Could you check a few things on this model? Use its own coordinates, in mm. A direction names the side the tool comes from. Round coordinates to 2 decimals unless told otherwise and drop trailing zeros. Order: outer loops, then holes, each group sorted by start corner. A loop starts at its lowest first (then second) coordinate and runs counter-clockwise, first axis right, second up. Notation, with made-up numbers: M 26,30 L 73,30 A18 ccw 73,45 Z; hole C -32,14.25 d11. An arc over 180 degrees is marked long. Write each question's results on one line, items separated by ' | '. Start each with the question number.
1. Suppose I cut it at A-A on z = 1.75. Write out the boundary of the cut face in (x, y).
2. Suppose I cut it at B-B on x = -16. Write out the boundary of the cut face in (y, z).
3. Suppose I cut it at C-C on y = 9. Write out the boundary of the cut face in (x, z), and give its area (3 significant figures).
4. Please list where these lines run through material, in increasing order: L1, parallel to X at y = 21, z = 2.5; L2, parallel to Z at x = 26.5, y = -8.5; L3, parallel to Y at x = 20, z = 2.25.
5. We'd pull the mould along X, two halves only. Please class faces 1 (the flat face through (-13.7, -27, 1)), 2 (the cylindrical face through (-6.525, -29.384, 1.986)), 3 (the cylindrical face through (2.9, 0, 5.1)), 4 (the flat face through (1.665, 17.4, 2.028)): released by +X, released by -X, zero draft, split by the parting line, or undercut.
6. For faces 5 (the flat face through (0, 2.05, 5)), 6 (the flat face through (-16.033, 6.961, 2.028)), 7 (the flat face through (-13.7, -27, 3)), 8 (the flat face through (0, -3, 9)), which set-ups out of +Z, -Z, +X, -X, +Y, -Y let a thin tool reach every point of the face, with its end or its side?
7. Suppose I cut it at D-D on z = 5.75. Write out the boundary of the cut face in (x, y), and give its area (3 significant figures).
8. I'm going to push flat-ended pins straight in: pin 1 (8 mm diameter, centred on x = -23.5, y = -8, fed in from +Z); pin 2 (1 mm diameter, centred on x = -12.5, z = 3.5, fed in from -Y); pin 3 (2 mm diameter, centred on x = 0.5, z = 3.5, fed in from -Y); pin 4 (10 mm diameter, centred on x = -6.5, y = 17.5, fed in from +Z). Where does each tip first touch, or does it pass through?
from build123d import *

# Parameters (mm, degrees)
F0_R      = 30.5
F1_DEPTH  = 4
F3_R      = 30.5
F3_R_2    = 30.1
F4_DEPTH  = 2
F5_R      = 5
F6_DEPTH  = 5
F8_DEPTH  = 8
F10_DEPTH = 25
F11_R     = 1


with BuildPart() as f1:
    # F0 (on Top) → F1 (new body)
    with BuildSketch(Plane.XY):
        Circle(F0_R)
    extrude(amount=F1_DEPTH)

    # F3 (on offset) → F4 (cut)
    with BuildSketch(Plane.XY.offset(1)):
        Circle(F3_R)
        Circle(F3_R_2, mode=Mode.SUBTRACT)
    extrude(amount=F4_DEPTH, mode=Mode.SUBTRACT)

    # F5 (on face) → F6 (join)
    with BuildSketch(Plane.XY.offset(4)):
        Circle(F5_R)
    extrude(amount=F6_DEPTH)

    # F7 (on face) → F8 (cut, through all)
    with BuildSketch(Plane.XY.offset(9)):
        with BuildLine():
            Line((2.0512191497, 2.05), (-2.0512191497, 2.05))
            ThreePointArc((-2.0512191497, 2.05), (-2.9, 0), (-2.0512191497, -2.05))
            Line((-2.0512191497, -2.05), (2.0512191497, -2.05))
            ThreePointArc((2.0512191497, -2.05), (2.9, 0), (2.0512191497, 2.05))
        make_face()
    extrude(amount=-F8_DEPTH, mode=Mode.SUBTRACT)

    # F9 (on face) → F10 (cut)
    with BuildSketch(Plane.XY.offset(4)):
        with BuildLine():
            Line((-3.3918327244, 10.4389877367), (6.8663471811, 24.5581610954))
            ThreePointArc((6.8663471811, 24.5581610954), (-7.8799333566, 24.2519411655), (-19.9899164741, 15.8320320667))
            Line((-19.9899164741, 15.8320320667), (-3.3918327244, 10.4389877367))
        make_face()
        with BuildLine():
            Line((8.8799333566, 6.4516492294), (25.4780171063, 1.0586048994))
            ThreePointArc((25.4780171063, 1.0586048994), (20.6299333566, 14.9885239335), (8.8799333566, 23.9039072869))
            Line((8.8799333566, 23.9039072869), (8.8799333566, 6.4516492294))
        make_face()
        with BuildLine():
            ThreePointArc((8.8799333566, -23.9039072869), (20.6299333566, -14.9885239335), (25.4780171063, -1.0586048994))
            Line((25.4780171063, -1.0586048994), (8.8799333566, -6.4516492294))
            Line((8.8799333566, -6.4516492294), (8.8799333566, -23.9039072869))
        make_face()
        with BuildLine():
            ThreePointArc((-19.9899164741, -15.8320320667), (-7.8799333566, -24.2519411655), (6.8663471811, -24.5581610954))
            Line((6.8663471811, -24.5581610954), (-3.3918327244, -10.4389877367))
            Line((-3.3918327244, -10.4389877367), (-19.9899164741, -15.8320320667))
        make_face()
        with BuildLine():
            Line((-10.9762012644, 0), (-21.2343811698, 14.1191733588))
            ThreePointArc((-21.2343811698, 14.1191733588), (-25.5, 0), (-21.2343811698, -14.1191733588))
            Line((-21.2343811698, -14.1191733588), (-10.9762012644, 0))
        make_face()
    extrude(amount=-F10_DEPTH, mode=Mode.SUBTRACT)

    # F11
    f11_edges = [f1.edges().sort_by_distance(p)[0] for p in [
        (-5, 0, 9),
        (-5, 0, 4),
    ]]
    fillet(f11_edges, radius=F11_R)


solid = f1.part
Filled sheet:
1) outline: C 0,0 d60.2; hole M -21.23,-14.12 L -10.98,0 L -21.23,14.12 A25.5 ccw Z; hole M -19.99,-15.83 A25.5 ccw 6.87,-24.56 L -3.39,-10.44 Z; hole M -19.99,15.83 L -3.39,10.44 L 6.87,24.56 A25.5 ccw Z; hole M -2.05,-2.05 L 2.05,-2.05 A2.9 ccw 2.05,2.05 L -2.05,2.05 A2.9 ccw Z; hole M 8.88,-23.9 A25.5 ccw 25.48,-1.06 L 8.88,-6.45 Z; hole M 8.88,6.45 L 25.48,1.06 A25.5 ccw 8.88,23.9 Z
2) outline: M -25.97,0 L -19.86,0 L -19.86,4 L -25.97,4 L -25.97,3 L -25.5,3 L -25.5,1 L -25.97,1 Z; M -14.54,0 L -6.91,0 L -6.91,4 L -14.54,4 Z; M 6.91,0 L 14.54,0 L 14.54,4 L 6.91,4 Z; M 19.86,0 L 25.97,0 L 25.97,1 L 25.5,1 L 25.5,3 L 25.97,3 L 25.97,4 L 19.86,4 Z
3) outline: M -29.14,0 L -23.86,0 L -23.86,4 L -29.14,4 L -29.14,3 L -28.72,3 L -28.72,1 L -29.14,1 Z; M -17.52,0 L 8.88,0 L 8.88,4 L -17.52,4 Z; M 23.86,0 L 29.14,0 L 29.14,1 L 28.72,1 L 28.72,3 L 29.14,3 L 29.14,4 L 23.86,4 Z | area: 146 mm^2
4) L1: x = -21.56 to -14.47, 4.28 to 8.88, 14.47 to 21.56 | L2: z = 0 to 4 | L3: y = -22.49 to -15.82, -2.84 to 2.84, 15.82 to 22.49
5) face 1: zero draft | face 2: split by the parting line | face 3: undercut | face 4: undercut
6) face 5: +Z | face 6: +Z, -Z | face 7: none | face 8: +Z, +X, -X, +Y, -Y
7) outline: C 0,0 d10; hole M -2.05,-2.05 L 2.05,-2.05 A2.9 ccw 2.05,2.05 L -2.05,2.05 A2.9 ccw Z | area: 56.9 mm^2
8) pin 1: stops at z = 4 | pin 2: stops at y = -28.04 | pin 3: stops at y = -30.5 | pin 4: passes through
